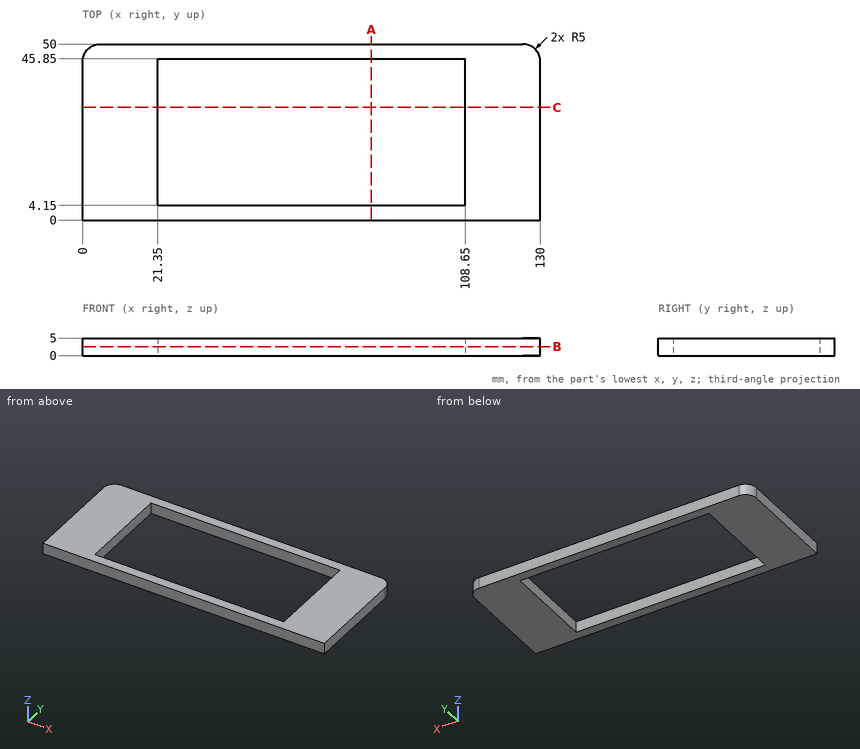
Source: three-view drawing plus pictorial views. Frame: mm from the lowest corner of the part. Round coordinates to 2 decimals unless told otherwise and drop trailing zeros. Order: outer loops, then holes, each group sorted by start corner. A loop starts at its lowest first (then second) coordinate and runs counter-clockwise, first axis right, second up. Notation, with made-up numbers: (66.5, 81.25) - (94.5, 81.25) arc R22 ccw to (94.5, 101.25) - close; hole circle Ø4 at (42, 77). An arc over 180 degrees is marked (long way). Answer in a Markdown table with one row per item.
Item 1: Section query A-A (x = 82). Return the cut outline in (y, z), then the cut area to 3 significant figures.
Model answer:
| item | result |
|---|---|
| outline | (0, 0) - (4.15, 0) - (4.15, 5) - (0, 5) - close; (45.85, 0) - (50, 0) - (50, 5) - (45.85, 5) - close |
| area | 41.5 mm² |
Item 2: Section query C-C (y = 32). Return the cut outline in (x, z), then the cut area to 4 significant figures.
Model answer:
| item | result |
|---|---|
| outline | (0, 0) - (21.35, 0) - (21.35, 5) - (0, 5) - close; (108.65, 0) - (130, 0) - (130, 5) - (108.65, 5) - close |
| area | 213.5 mm² |
Item 3: Line query: line 1 (X direction, y = 19, z = 1.35); line 2 (Y direction, x = 33, z = 4.85). Output: solid intervals per line, ascending.
Model answer:
| item | result |
|---|---|
| line 1 | x = 0 to 21.35, 108.65 to 130 |
| line 2 | y = 0 to 4.15, 45.85 to 50 |
Item 4: Section query B-B (z = 2.6). Return the cut outline in (x, y).
Model answer:
| item | result |
|---|---|
| outline | (0, 0) - (130, 0) - (130, 45) arc R5 ccw to (125, 50) - (5, 50) arc R5 ccw to (0, 45) - close; hole (21.35, 4.15) - (108.65, 4.15) - (108.65, 45.85) - (21.35, 45.85) - close |
